Autodesk Fusion 360 part; units mm, degrees
sketch "Sketch1" plane through (0, 0, 0) normal (0, 1, 0) x (1, 0, 0)
  circle A0 centre (0, 0) radius 150
  circle A1 centre (-36.4232, 65.5618) radius 11.5
  circle A2 centre (-36.4232, 65.5618) radius 17.5
  circle A3 centre (-65.5618, -36.4232) radius 17.5
  circle A4 centre (-65.5618, -36.4232) radius 11.5
  circle A5 centre (36.4232, -65.5618) radius 17.5
  circle A6 centre (36.4232, -65.5618) radius 11.5
  circle A7 centre (65.5618, 36.4232) radius 17.5
  circle A8 centre (65.5618, 36.4232) radius 11.5
  circle A9 centre (0, 0) radius 35
  circle A10 centre (0, 0) radius 40.15
  circle A11 centre (0, 0) radius 43.5
  circle A12 centre (0, 0) radius 97.5
  line L0 (0, 0) -> (169.7056, 0) construction
  circle A13 centre (-89.8026, 89.8026) radius 11.75
  circle A14 centre (-89.8026, -89.8026) radius 11.75
  circle A15 centre (89.8026, -89.8026) radius 11.75
  circle A16 centre (89.8026, 89.8026) radius 11.75
  circle A17 centre (-62.8594, 56.9974) radius 6
  dimension "d13" = 300
  dimension "d17" = 23
  dimension "d18" = 35
  dimension "d21" = 70
  dimension "d22" = 80.3
  dimension "d23" = 87
  dimension "d24" = 195
  dimension "d26" = 23.5
  dimension "d28" = 360
  dimension "d31" = 12
extrude "Extrude1" add sketch "Sketch1" along normal blind 40 contours A10 makes body 1
extrude "Extrude2" add sketch "Sketch1" along normal blind 38 contours A11 | A12 bodies 1
extrude "Extrude3" add sketch "Sketch1" along normal blind 30 contours A0 bodies 1
extrude "Extrude4" add sketch "Sketch1" along normal blind 5 separate body contours A10 | A11 makes body 2
combine "Combine1" operation cut target body 1 tool bodies 2
extrude "Extrude5" add sketch "Sketch1" along normal blind 14 separate body contours A2 | A3 | A5 | A7 makes body 3 at (83.04, 4.6667, -35.5509) makes body 4 at (-48.0835, 4.6667, 37.2955) makes body 5 at (-18.945, 4.6667, -64.6895) makes body 6 at (53.8363, 9.3333, 67.3042)
combine "Combine2" operation add target body 1 tool bodies 3 5 4 6
scale "Scale1" factor 0.2 about (-35, 5, 0) bodies 1
scale "Scale2" factor 1.5 about (-35, 5, 0) bodies 1
Check sheet for the modelled part. Datum: model origin and axes. Units: mm. A direction names the side the tool comes from. Round coordinates to 2 decimals unless told otherwise and drop trailing zeros. Order: outer loops, then holes, each group sorted by start corner. A loop starts at its lowest first (then second) coordinate and runs counter-clockwise, first axis right, second up.
(1) Cross-section at D-D, the plane x = -63. Enter the section's corners in (y, z), and give its area (3 significant figures).
(2) Cross-section at B-B, the plane x = -25. Enter the section's corners in (y, z).
(3) Cross-section at C-C, the plane y = 9.5. State how many separate pieces and enclosed holes the cut face has, and give its area (3 significant figures).
(4) Scan lines: probe 1 along X at (y, z) = (9.5, 15); probe 2 along X at (y, z) = (4.5, -18); probe 3 along Z at (x, y) = (-15.5, 14). Record each from-to range of solid material in increasing order.
(5) Cross-section at A-A, the plane z = 0. Enter the section's corners in (x, y) (3 decimals), and give its area (3 significant figures).
(6) Go/stop test with flat-tipped pins: P1, Ø5, axis at y = 13.5, z = -10, coming from the -X side; P2, Ø3, axis at x = -37, z = -20.5, coming from the +Y side; P3, Ø4.5, axis at x = -43.36, z = -17.1, coming from the -Y side; P4, Ø12, axis at x = 8, z = 22, coming from the +Y side. Record where each tip stops, or that it passes through.
(7) Draft check along X on faces 1 (the flat face through (-12, 14.9, 0)), 2 (the cylindrical face through (-12.053, 4.24, 3.92)), 3 (the cylindrical face through (-30.841, 13.683, -28.554)). Enter one of: pulls with the +X half, pulls with the -X half, needs draft (parallel to the pull), parting line crosses it, or undercut.
(8) Access from +Z, -Z, +X, -X, +Y, -Y to the whole of each face (thin tool, end or side, straight path). Record for faces 4 (the flat face through (-3.7, 7.7, -7.5)), 5 (the cylindrical face through (-5.579, 5.571, -14.295)).
Check sheet entries:
1. outline: (3.5, -23.3) - (12.5, -23.3) - (12.5, 23.3) - (3.5, 23.3) - close
1. area: 419 mm2
2. outline: (3.5, -45) - (12.5, -45) - (12.5, -29.25) - (14.9, -29.25) - (14.9, -12.03) - (15.5, -12.03) - (15.5, -10.49) - (5, -10.49) - (5, -13.04) - (3.5, -13.04) - close; (3.5, 13.04) - (5, 13.04) - (5, 10.49) - (15.5, 10.49) - (15.5, 12.03) - (14.9, 12.03) - (14.9, 29.25) - (12.5, 29.25) - (12.5, 45) - (3.5, 45) - close
3. separate pieces: 1
3. enclosed holes: 10
3. area: 5,500 mm2
4. probe 1: x = -66.93 to -47.48, -40.86 to -15.97, -11.17 to 17.93
4. probe 2: x = -65.74 to -44.92, -41.8 to -38.45, -32.41 to 16.74
4. probe 3: z = -27.83 to -5.41, 5.41 to 14.78, 24.55 to 27.83
5. outline: (-69.5, 3.5) - (-37.55, 3.5) - (-37.55, 5) - (-35, 5) - (-35, 15.5) - (-36.545, 15.5) - (-36.545, 14.9) - (-53.75, 14.9) - (-53.75, 12.5) - (-69.5, 12.5) - close; (-14, 5) - (-11.45, 5) - (-11.45, 3.5) - (20.5, 3.5) - (20.5, 12.5) - (4.75, 12.5) - (4.75, 14.9) - (-12.455, 14.9) - (-12.455, 15.5) - (-14, 15.5) - close
5. area: 705 mm2
6. P1: stops at x = -68.83
6. P2: passes through
6. P3: stops at y = 3.5
6. P4: stops at y = 12.5
7. face 1: needs draft
7. face 2: undercut
7. face 3: parting line crosses it
8. face 4: +Y
8. face 5: +Y, -Y
